The model under review builds one solid part; all positions refer to its coordinate system, in mm. A direction names the side the tool comes from. Coordinates: 2 decimals unless noted, no trailing zeros. Loops run counter-clockwise (first coordinate to the right, second up) from the corner with the lowest first, then second, coordinate; pieces in that order, holes last. Notation, with made-up numbers: (26, 25) -> (75, 25) arc R19 cw to (75, 48) -> close; hole circle Ø5 at (-7, 62.5). An arc over 180 degrees is marked (long way). One line per question, with ' | ' between items. Start each with the question number.
from build123d import *
from OCP.BRepFilletAPI import BRepFilletAPI_MakeChamfer

# Parameters (mm, degrees)
EXTRUDE_1_DEPTH     = 30
EXTRUDE_2_DEPTH     = 14
SKETCH_3_W          = 0.1
SKETCH_3_H          = 0.1
CUT_EXTRUDE_1_DEPTH = 12
CHAMFER_1_SIZE      = 4.367642811
CHAMFER_1_SIZE_2    = 12


with BuildPart() as part:
    # ｽｹｯﾁ1 → ﾎﾞｽ - 押し出し1 (new body)
    with BuildSketch(Plane(origin=(0, 0, 0), x_dir=(1, 0, 0), z_dir=(0, 1, 0))):
        Polygon((3.464101615, -6), (6.92820323, 0), (3.464101615, 6), (-3.464101615, 6), (-6.92820323, 0), (-3.464101615, -6), align=None)
    extrude(amount=EXTRUDE_1_DEPTH)

    # ｽｹｯﾁ2 → ﾎﾞｽ - 押し出し2 (add)
    with BuildSketch(Plane(origin=(0, 30, 0), x_dir=(1, 0, 0), z_dir=(0, 1, 0))):
        Polygon((6.350852961, -11), (12.701705922, 0), (6.350852961, 11), (-6.350852961, 11), (-12.701705922, 0), (-6.350852961, -11), align=None)
    extrude(amount=EXTRUDE_2_DEPTH)

    # ｽｹｯﾁ3 → ｶｯﾄ - 押し出し1 (cut)
    with BuildSketch(Plane(origin=(0, 44, 0), x_dir=(1, 0, 0), z_dir=(0, 1, 0))):
        Rectangle(SKETCH_3_W, SKETCH_3_H)
    extrude(amount=-CUT_EXTRUDE_1_DEPTH, mode=Mode.SUBTRACT)

    # 面取り1
    chamfer_1_edges_1 = [part.edges().sort_by_distance(p)[0] for p in [
        (0, 44, 0.05),
    ]]
    chamfer_1_side_1 = [part.faces().sort_by_distance(p)[0] for p in [
        (0, 44, 0.137352856),
    ]]
    chamfer_1_edges_2 = [part.edges().sort_by_distance(p)[0] for p in [
        (-0.05, 44, 0),
    ]]
    chamfer_1_side_2 = [part.faces().sort_by_distance(p)[0] for p in [
        (-0.137352856, 44, 0),
    ]]
    chamfer_1_edges_3 = [part.edges().sort_by_distance(p)[0] for p in [
        (0, 44, -0.05),
    ]]
    chamfer_1_side_3 = [part.faces().sort_by_distance(p)[0] for p in [
        (0, 44, -0.137352856),
    ]]
    chamfer_1_edges_4 = [part.edges().sort_by_distance(p)[0] for p in [
        (0.05, 44, 0),
    ]]
    chamfer_1_side_4 = [part.faces().sort_by_distance(p)[0] for p in [
        (0.137352856, 44, 0),
    ]]
    chamfer_1 = BRepFilletAPI_MakeChamfer(part.part.solid().wrapped)
    for e in chamfer_1_edges_1:
        chamfer_1.Add(CHAMFER_1_SIZE - 0.0001, CHAMFER_1_SIZE_2 - 0.0001, e.wrapped, chamfer_1_side_1[0].wrapped)
    for e in chamfer_1_edges_2:
        chamfer_1.Add(CHAMFER_1_SIZE - 0.0001, CHAMFER_1_SIZE_2 - 0.0001, e.wrapped, chamfer_1_side_2[0].wrapped)
    for e in chamfer_1_edges_3:
        chamfer_1.Add(CHAMFER_1_SIZE - 0.0001, CHAMFER_1_SIZE_2 - 0.0001, e.wrapped, chamfer_1_side_3[0].wrapped)
    for e in chamfer_1_edges_4:
        chamfer_1.Add(CHAMFER_1_SIZE - 0.0001, CHAMFER_1_SIZE_2 - 0.0001, e.wrapped, chamfer_1_side_4[0].wrapped)
    add(Compound.cast(chamfer_1.Shape()), mode=Mode.REPLACE)  # a hair under: the kernel refuses the full size


solid = part.part
1) Wall thickness on L1, parallel to Z at x = 1, y = 15.5; L2, parallel to Y at x = 7.25, z = -4.5; L3, parallel to X at y = 32, z = -2.5: over which ranges is each line inside the solid? List them lowest first.
2) Consider section C-C, the plane z = -1. Write out the cut boundary in (x, y), plus the area to 3 significant figures.
3) Consider section D-D, the plane y = 16. Write out the cut boundary in (x, z).
4) Insertion check: pin 1 Ø8 at (y, z) = (15.5, -6) entering from +X; pin 2 Ø7.5 at (x, y) = (-1, 20.5) entering from -Z; pin 3 Ø8 at (x, y) = (-3.5, 17) entering from +Z. Each pin has a flat end and moves straight along its axis. Give the tip position at first contact, or say it passes through.
5) Mouldability with a two-part tool opening along X and no side actions: class faces 5 (the face through (-5.22, 14.79, 2.96)), 6 (the face through (-0.06, 39.25, -2.69)), 7 (the face through (0, 15, 6)) as +X half, -X half, draft (parallel to the pull), parting line (faces both ways), or undercut.
6) Consider section B-B, the plane x = -5. Write out the cut boundary in (y, z).
7) Machinability: for faces 1 (the face through (5, 30, -5)), 2 (the face through (-2.69, 39.25, 0.06)), 3 (the face through (0, 15, -6)), 4 (the face through (-5.172, 14.79, -3.042)), which of the approach directions +Z, -Z, +X, -X, +Y, -Y give a long, thin tool a straight path to every point of the face, cutting with its end or side? Answer none if there is none.
8) Consider section A-A, the plane y = 39. Write out the cut boundary in (x, z), plus the area to 3 significant figures.
Filled sheet:
1) L1: -6 to 6 | L2: 30 to 44 | L3: -11.26 to 11.26
2) outline: (-12.12, 30) -> (-6.35, 30) -> (-6.35, 0) -> (6.35, 0) -> (6.35, 30) -> (12.12, 30) -> (12.12, 44) -> (4.42, 44) -> (1, 34.61) -> (-1, 34.61) -> (-4.42, 44) -> (-12.12, 44) -> close | area: 670 mm^2
3) outline: (-6.93, 0) -> (-3.46, -6) -> (3.46, -6) -> (6.93, 0) -> (3.46, 6) -> (-3.46, 6) -> close
4) pin 1: x = 5.77 | pin 2: z = -6 | pin 3: z = 6
5) face 5: -X half | face 6: undercut | face 7: draft
6) outline: (0, -3.34) -> (30, -3.34) -> (30, -11) -> (44, -11) -> (44, 11) -> (30, 11) -> (30, 3.34) -> (0, 3.34) -> close
7) face 1: -Y | face 2: +Y | face 3: -Z, +X, -X, -Y | face 4: -Z, -X, -Y
8) outline: (-12.7, 0) -> (-6.35, -11) -> (6.35, -11) -> (12.7, 0) -> (6.35, 11) -> (-6.35, 11) -> close; hole (-2.6, -2.6) -> (2.6, -2.6) -> (2.6, 2.6) -> (-2.6, 2.6) -> close | area: 392 mm^2
